from build123d import *

# Parameters (mm, degrees)
SKETCH1_W            = 8.2
SKETCH1_H            = 4
BOSS_EXTRUDE1_DEPTH  = 4
FILLET1_R            = 1
FILLET1_OF_MIRROR1_R = 1


with BuildPart() as part:
    # Sketch1 → Boss-Extrude1 (new body)
    with BuildSketch(Plane(origin=(0, 0, 0), x_dir=(1, 0, 0), z_dir=(0, 1, 0))):
        Polygon((0, 52.3), (0, 0), (13.36, 0), (13.36, 11.1), (19.5, 11.1), (19.5, 29.1), (47, 29.1), (47, 52.3), (34.5, 52.3), (34.5, 56.3), (47, 56.3), (47, 59.7), (29.5, 59.7), (29.5, 48.3), (13.36, 48.3), (13.36, 52.3), align=None)
        with Locations((6.68, 5)):
            Rectangle(SKETCH1_W, SKETCH1_H, mode=Mode.SUBTRACT)
    boss_extrude1 = extrude(amount=BOSS_EXTRUDE1_DEPTH)

    # Fillet1
    fillet1_edges = [part.edges().sort_by_distance(p)[0] for p in [
        (19.5, 2, -29.1),
        (13.36, 2, 0),
        (0, 2, 0),
        (29.5, 2, -59.7),
    ]]
    fillet(fillet1_edges, radius=FILLET1_R)

    # Mirror1: Boss-Extrude1 across plane
    add(boss_extrude1.mirror(Plane(origin=(47, 4, 0), x_dir=(0, 0, 1), z_dir=(1, 0, 0))))

    # Fillet1 of Mirror1
    fillet1_of_mirror1_edges = [part.edges().sort_by_distance(p)[0] for p in [
        (74.5, 2, -29.1),
        (80.64, 2, 0),
        (94, 2, 0),
        (64.5, 2, -59.7),
    ]]
    fillet(fillet1_of_mirror1_edges, radius=FILLET1_OF_MIRROR1_R)


solid = part.part
The model under review builds one solid part; all positions refer to its coordinate system, in mm. A direction names the side the tool comes from. Give positions to 0.01 mm unless a question says otherwise; leave off trailing zeros. Order: outer loops, then holes, each group sorted by start corner. A loop starts at its lowest first (then second) coordinate and runs counter-clockwise, first axis right, second up. Notation, with made-up numbers: (41.5, 54.5) -> (86.5, 54.5) arc R25 cw to (86.5, 67.5) -> close; hole circle Ø5 at (64.25, 54). An arc over 180 degrees is marked (long way). Write item = value, one per line. Start each with the question number.
(1) Tool access review of faces 1 (the flat face through (13.36, 2, -50)), 2 (the flat face through (80.64, 2, -6)), 3 (the flat face through (2.58, 2, -5)), 4 (the flat face through (87, 2, -52.3)), 5 (the flat face through (7, 2, 0)): name each direction out of +Z, -Z, +X, -X, +Y, -Y from which nothing blocks a thin tool from reaching the whole face with its end or side.
(2) Take a section at A-A (z = -23). Write out the cut boundary in (x, y), plus the area to 3 significant figures.
(3) Take a section at B-B (x = 8). Write out the cut boundary in (y, z).
(4) For pin 1 Ø2 at (y, z) = (1, -55) entering from -X; pin 2 Ø1.2 at (x, y) = (8.5, 2) entering from -Z, all flat-tipped, find the tip position at first contact; note any pin that passes through.
(5) For L1, parallel to X at y = 2.25, z = -53.5; L2, parallel to X at y = 0.9, z = -25.5; L3, parallel to Z at x = 39.5, y = 2, list the stretches that pass through material, from the lowest coordinate up. Write a range as from..to.
(6) Draft analysis for pull direction Z (two halves, no side actions). For faces 6 (the flat face through (29.5, 2, -54)), 7 (the flat face through (87, 2, -7)), 8 (the flat face through (16, 2, -11.1)), state which applies: +Z half, -Z half, draft (parallel to the pull), parting line (faces both ways), or undercut.
(7) Take a section at D-D (y = 1.35). State how many separate pieces and enclosed holes the cut face has, plus the area to 3 significant figures.
(8) Take a section at C-C (x = 23). Write out the cut boundary in (y, z).
Returned:
q1.face_1 = -Z, +Y, -Y
q1.face_2 = +Z, +Y, -Y
q1.face_3 = +Y, -Y
q1.face_4 = -Z, +X, +Y, -Y
q1.face_5 = +Z, +X, -X, +Y, -Y
q2.outline = (0, 0) -> (19.5, 0) -> (19.5, 4) -> (0, 4) -> close; (74.5, 0) -> (94, 0) -> (94, 4) -> (74.5, 4) -> close
q2.area = 156 mm²
q3.outline = (0, -52.3) -> (4, -52.3) -> (4, -7) -> (0, -7) -> close; (0, -3) -> (4, -3) -> (4, 0) -> (0, 0) -> close
q4.pin_1 = 29.5
q4.pin_2 = -52.3
q5.L1 = 29.5..34.5, 59.5..64.5
q5.L2 = 0..19.5, 74.5..94
q5.L3 = -59.7..-56.3, -52.3..-29.1
q6.face_6 = draft
q6.face_7 = undercut
q6.face_8 = +Z half
q7.separate_pieces = 1
q7.enclosed_holes = 3
q7.area = 3,140 mm²
q8.outline = (0, -48.3) -> (4, -48.3) -> (4, -29.1) -> (0, -29.1) -> close
